Design review of the part built by this model. Coordinates are the model's own, in mm. Face numbers are marked on the shaded views. A direction names the side the tool comes from. Round coordinates to 2 decimals unless told otherwise and drop trailing zeros. Write each loop counter-clockwise with the first axis right and the second up, starting at its lowest first coordinate (ties: lowest second). Pieces come first, ordered by that corner, then holes. Notation, with made-up numbers: M 75.5,27 L 80.5,27 A8 cw 80.5,33 Z; hole C 9.25,59.25 d8. An arc over 180 degrees is marked long. One line per question, with ' | ' between items. Start each with the question number.
Item 1: Draft analysis for pull direction Y (two halves, no side actions). For the marked faces 1, 2 and 3, state which applies: released by +Y, released by -Y, zero draft, split by the parting line, or undercut.
Item 2: Machinability: for the marked faces 4, 5, 6 and 7, which of the approach directions +Z, -Z, +X, -X, +Y, -Y give a long, thin tool a straight path to every point of the face, cutting with its end or side? Answer none if there is none.
Item 3: Add section B-B, the plane y = 40. State the section outline as (x, z) points, and give its area (3 significant figures).
Item 4: For L1, parallel to X at y = 16, z = 5; L2, parallel to Y at x = 26, z = 5; L3, parallel to X at y = 15, z = 9.5, list the stretches that pass through material, from the lowest coordinate up.
Item 5: Add section C-C, the plane x = -35. State the section outline as (y, z) points.
Item 6: Insertion check: pin 1 Ø1.4 at (x, y) = (25.5, 21) entering from +Z; pin 2 Ø1.7 at (x, y) = (67, -26) entering from +Z; pin 3 Ø5 at (x, y) = (64, -26) entering from +Z. Each pin has a flat end and moves straight along its axis. Give the tip position at first contact, or say it passes through.
Item 7: Add section A-A, the plane z = 6. Give the number of separate pieces and of enclosed holes in the cut face, and give its area (3 significant figures).
```python
from build123d import *

# Parameters (mm, degrees)
SKETCH_W             = 112
SKETCH_H             = 62
PAD_DEPTH            = 45
THICKNESS_T          = -2
SKETCH001_R          = 4
SKETCH001_R_2        = 1.45
PAD001_DEPTH         = 9
POCKET_DEPTH         = 5
POCKET001_DEPTH      = 31.001
POCKET001_DEPTH_BACK = 31.001
SKETCH004_W          = 15
SKETCH004_H          = 8
POCKET002_DEPTH      = 72.001
SKETCH005_W          = 15
SKETCH005_H          = 8
SKETCH005_W_2        = 2.5
SKETCH005_H_2        = 4
POCKET003_DEPTH      = 40.001
PAD002_DEPTH         = 43
SKETCH007_R          = 1.45
POCKET004_DEPTH      = 10
SKETCH009_W          = 20
SKETCH009_H          = 20
SKETCH009_R          = 2.75
PAD004_DEPTH         = 6


with BuildPart() as part:
    # Sketch → Pad (new body)
    with BuildSketch(Plane.XY):
        with Locations((16, 0)):
            Rectangle(SKETCH_W, SKETCH_H)
    extrude(amount=PAD_DEPTH)

    # Thickness
    thickness_openings = [part.faces().sort_by_distance(p)[0] for p in [
        (16, 0, 45),
    ]]
    offset(amount=THICKNESS_T, openings=thickness_openings, kind=Kind.INTERSECTION)

    # Sketch001 → Pad001 (join)
    with BuildSketch(Plane.XY):
        with Locations((-26, 21)):
            Circle(SKETCH001_R)
        with Locations((-26, 21)):
            Circle(SKETCH001_R_2, mode=Mode.SUBTRACT)
        with Locations((26, 21)):
            Circle(SKETCH001_R)
        with Locations((26, 21)):
            Circle(SKETCH001_R_2, mode=Mode.SUBTRACT)
        with Locations((-26, -21)):
            Circle(SKETCH001_R)
        with Locations((-26, -21)):
            Circle(SKETCH001_R_2, mode=Mode.SUBTRACT)
        with Locations((26, -21)):
            Circle(SKETCH001_R)
        with Locations((26, -21)):
            Circle(SKETCH001_R_2, mode=Mode.SUBTRACT)
        with Locations((62.5, 16)):
            Circle(SKETCH001_R)
        with Locations((62.5, 16)):
            Circle(SKETCH001_R_2, mode=Mode.SUBTRACT)
        with Locations((45, -16)):
            Circle(SKETCH001_R)
        with Locations((45, -16)):
            Circle(SKETCH001_R_2, mode=Mode.SUBTRACT)
    extrude(amount=PAD001_DEPTH)

    # Sketch002 → Pocket (cut)
    with BuildSketch(Plane.XY):
        with BuildLine():
            ThreePointArc((-28, 14.5), (-30.5, 12), (-28, 9.5))
            Line((-28, 9.5), (32, 9.5))
            ThreePointArc((32, 9.5), (34.5, 12), (32, 14.5))
            Line((32, 14.5), (-28, 14.5))
        make_face()
        with BuildLine():
            ThreePointArc((-28, 6.5), (-30.5, 4), (-28, 1.5))
            Line((-28, 1.5), (32, 1.5))
            ThreePointArc((32, 1.5), (34.5, 4), (32, 6.5))
            Line((32, 6.5), (-28, 6.5))
        make_face()
        with BuildLine():
            ThreePointArc((-28, -1.5), (-30.5, -4), (-28, -6.5))
            Line((-28, -6.5), (32, -6.5))
            ThreePointArc((32, -6.5), (34.5, -4), (32, -1.5))
            Line((32, -1.5), (-28, -1.5))
        make_face()
        with BuildLine():
            ThreePointArc((-28, -9.5), (-30.5, -12), (-28, -14.5))
            Line((-28, -14.5), (32, -14.5))
            ThreePointArc((32, -14.5), (34.5, -12), (32, -9.5))
            Line((32, -9.5), (-28, -9.5))
        make_face()
    extrude(amount=POCKET_DEPTH, mode=Mode.SUBTRACT)

    # Sketch003 → Pocket001 (cut, two sides)
    with BuildSketch(Plane.XZ) as pocket001_sk:
        with BuildLine():
            ThreePointArc((-18, 37.5), (-20.5, 35), (-18, 32.5))
            Line((-18, 32.5), (12, 32.5))
            ThreePointArc((12, 32.5), (14.5, 35), (12, 37.5))
            Line((12, 37.5), (-18, 37.5))
        make_face()
        with BuildLine():
            ThreePointArc((-18, 27.5), (-20.5, 25), (-18, 22.5))
            Line((-18, 22.5), (12, 22.5))
            ThreePointArc((12, 22.5), (14.5, 25), (12, 27.5))
            Line((12, 27.5), (-18, 27.5))
        make_face()
        with BuildLine():
            ThreePointArc((-18, 17.5), (-20.5, 15), (-18, 12.5))
            Line((-18, 12.5), (12, 12.5))
            ThreePointArc((12, 12.5), (14.5, 15), (12, 17.5))
            Line((12, 17.5), (-18, 17.5))
        make_face()
        with BuildLine():
            ThreePointArc((37, 37.5), (34.5, 35), (37, 32.5))
            Line((37, 32.5), (55, 32.5))
            ThreePointArc((55, 32.5), (57.5, 35), (55, 37.5))
            Line((55, 37.5), (37, 37.5))
        make_face()
        with BuildLine():
            ThreePointArc((37, 27.5), (34.5, 25), (37, 22.5))
            Line((37, 22.5), (55, 22.5))
            ThreePointArc((55, 22.5), (57.5, 25), (55, 27.5))
            Line((55, 27.5), (37, 27.5))
        make_face()
        with BuildLine():
            ThreePointArc((37, 17.5), (34.5, 15), (37, 12.5))
            Line((37, 12.5), (55, 12.5))
            ThreePointArc((55, 12.5), (57.5, 15), (55, 17.5))
            Line((55, 17.5), (37, 17.5))
        make_face()
    extrude(amount=-POCKET001_DEPTH, mode=Mode.SUBTRACT)
    extrude(pocket001_sk.sketch, amount=POCKET001_DEPTH_BACK, mode=Mode.SUBTRACT)

    # Sketch004 → Pocket002 (cut, through all)
    with BuildSketch(Plane.YZ):
        with Locations((20.5, 29)):
            Rectangle(SKETCH004_W, SKETCH004_H)
    extrude(amount=POCKET002_DEPTH, mode=Mode.SUBTRACT)

    # Sketch005 → Pocket003 (cut, through all)
    with BuildSketch(Plane.YZ):
        with Locations((-11, 28)):
            Rectangle(SKETCH005_W, SKETCH005_H)
        with Locations((11, 28)):
            Rectangle(SKETCH005_W, SKETCH005_H)
        with Locations((-17.25, 38)):
            Rectangle(SKETCH005_W_2, SKETCH005_H_2)
        with Locations((-4.75, 38)):
            Rectangle(SKETCH005_W_2, SKETCH005_H_2)
        with Locations((4.75, 38)):
            Rectangle(SKETCH005_W_2, SKETCH005_H_2)
        with Locations((17.25, 38)):
            Rectangle(SKETCH005_W_2, SKETCH005_H_2)
        with Locations((-17.25, 18)):
            Rectangle(SKETCH005_W_2, SKETCH005_H_2)
        with Locations((-4.75, 18)):
            Rectangle(SKETCH005_W_2, SKETCH005_H_2)
        with Locations((4.75, 18)):
            Rectangle(SKETCH005_W_2, SKETCH005_H_2)
        with Locations((17.25, 18)):
            Rectangle(SKETCH005_W_2, SKETCH005_H_2)
    extrude(amount=-POCKET003_DEPTH, mode=Mode.SUBTRACT)

    # Sketch006 → Pad002 (join)
    with BuildSketch(Plane.XY):
        Polygon((-38, 29), (-28, 29), (-38, 19), align=None)
        Polygon((70, -29), (70, -19), (60, -29), align=None)
    extrude(amount=PAD002_DEPTH)

    # Sketch007 (on DatumPlane) → Pocket004 (cut)
    with BuildSketch(Plane.XY.offset(43)):
        with Locations((-35, 26)):
            Circle(SKETCH007_R)
        with Locations((67, -26)):
            Circle(SKETCH007_R)
    extrude(amount=-POCKET004_DEPTH, mode=Mode.SUBTRACT)

    # Sketch009 (on DatumPlane) → Pad004 (join)
    with BuildSketch(Plane.XY.offset(38)):
        with Locations((-30, 40)):
            Rectangle(SKETCH009_W, SKETCH009_H)
        with Locations((-30, 40)):
            Circle(SKETCH009_R, mode=Mode.SUBTRACT)
        with Locations((62, 40)):
            Rectangle(SKETCH009_W, SKETCH009_H)
        with Locations((62, 40)):
            Circle(SKETCH009_R, mode=Mode.SUBTRACT)
    extrude(amount=PAD004_DEPTH)


solid = part.part
```
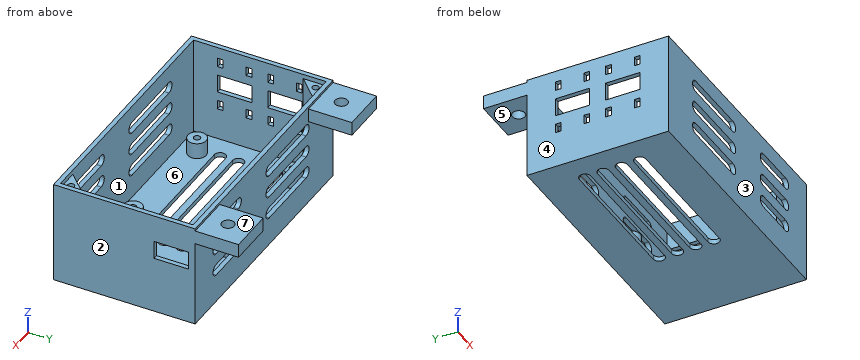
Computed values:
1) face 1: undercut | face 2: zero draft | face 3: released by -Y
2) face 4: +Z, -Z, -X, +Y, -Y | face 5: -Z, +X, -X, +Y | face 6: +Z | face 7: +Z, +X, -X, +Y
3) outline: M -40,38 L -32.75,38 L -32.75,44 L -40,44 Z; M -27.25,38 L -20,38 L -20,44 L -27.25,44 Z; M 52,38 L 59.25,38 L 59.25,44 L 52,44 Z; M 64.75,38 L 72,38 L 72,44 L 64.75,44 Z | area: 174 mm^2
4) L1: x = -40 to -38, 58.5 to 61.05, 63.95 to 66.5, 70 to 72 | L2: y = -31 to -29, -25 to -22.45, -19.55 to -17, 17 to 19.55, 22.45 to 25, 29 to 31 | L3: x = -40 to -38, 70 to 72
5) outline: M -31,0 L 31,0 L 31,38 L 50,38 L 50,44 L 31,44 L 31,45 L 29,45 L 29,43 L 27.45,43 L 27.45,33 L 24.55,33 L 24.55,43 L 22,43 L 22,2 L -29,2 L -29,45 L -31,45 Z
6) pin 1: stops at z = 2 | pin 2: stops at z = 33 | pin 3: stops at z = 43
7) separate pieces: 7 | enclosed holes: 7 | area: 1,040 mm^2
